```python
from build123d import *

# Parameters (mm, degrees)
SKETCH1_W           = 6.3
SKETCH1_H           = 8
SKETCH1_R           = 1.75
BOSS_EXTRUDE1_DEPTH = 10
SKETCH2_W           = 20
SKETCH2_H           = 6.3
SKETCH2_R           = 1.75
BOSS_EXTRUDE2_DEPTH = 12.15
SKETCH3_R           = 1.325
CUT_EXTRUDE1_DEPTH  = 31.009081959
SKETCH4_W           = 8.6
SKETCH4_H           = 6.3
CUT_EXTRUDE2_DEPTH  = 10
CUT_EXTRUDE3_DEPTH  = 31.009081959
SKETCH13_W          = 5.8
SKETCH13_H          = 3
CUT_EXTRUDE4_DEPTH  = 26.106025173


with BuildPart() as part:
    # Sketch1 → Boss-Extrude1 (new body)
    with BuildSketch(Plane(origin=(0, 0, 0), x_dir=(0, 1, 0), z_dir=(0, 0, 1))):
        Rectangle(SKETCH1_W, SKETCH1_H)
        with Locations(Location((0, 0, 0), (0, 0, 270))):
            Circle(SKETCH1_R, mode=Mode.SUBTRACT)
    extrude(amount=BOSS_EXTRUDE1_DEPTH)

    # Sketch2 → Boss-Extrude2 (add)
    with BuildSketch(Plane.XY.offset(10)):
        Rectangle(SKETCH2_W, SKETCH2_H)
        Circle(SKETCH2_R, mode=Mode.SUBTRACT)
    extrude(amount=BOSS_EXTRUDE2_DEPTH)

    # Sketch3 → Cut-Extrude1 (cut, through all)
    with BuildSketch(Plane(origin=(-10, 0, 0), x_dir=(0, -1, 0), z_dir=(-1, 0, 0))):
        with Locations(Location((0, 19, 0), (0, 0, 90))):
            Circle(SKETCH3_R)
    extrude(amount=-CUT_EXTRUDE1_DEPTH, mode=Mode.SUBTRACT)

    # Sketch4 → Cut-Extrude2 (cut)
    with BuildSketch(Plane.XY.offset(22.15)):
        Rectangle(SKETCH4_W, SKETCH4_H)
    extrude(amount=-CUT_EXTRUDE2_DEPTH, mode=Mode.SUBTRACT)

    # Sketch11 → Cut-Extrude3 (cut, through all)
    with BuildSketch(Plane(origin=(-10, 0, 0), x_dir=(0, -1, 0), z_dir=(-1, 0, 0))):
        with BuildLine():
            Line((-3.15, 19), (-3.15, 24.112369899))
            Line((-3.15, 24.112369899), (3.15, 24.112369899))
            Line((3.15, 24.112369899), (3.15, 19))
            ThreePointArc((3.15, 19), (0, 22.15), (-3.15, 19))
        make_face()
    extrude(amount=-CUT_EXTRUDE3_DEPTH, mode=Mode.SUBTRACT)

    # Sketch13 → Cut-Extrude4 (cut, through all)
    with BuildSketch(Plane(origin=(0, 3.15, 0), x_dir=(-1, 0, 0), z_dir=(0, 1, 0))):
        with Locations((0, 3)):
            Rectangle(SKETCH13_W, SKETCH13_H)
    extrude(amount=-CUT_EXTRUDE4_DEPTH, mode=Mode.SUBTRACT)


solid = part.part
```
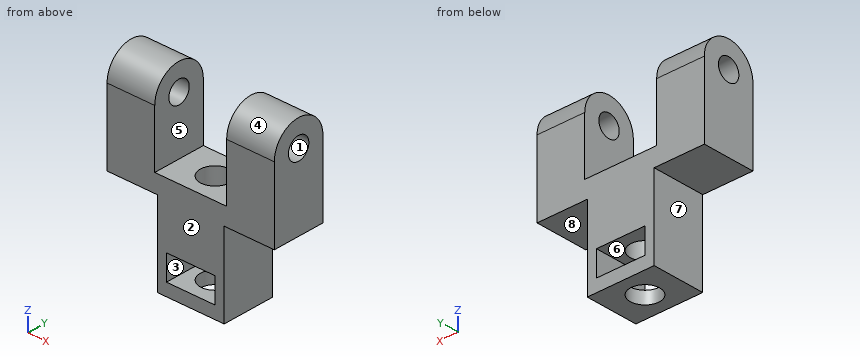
For this review, take the finished solid that the model builds, in its own axes (mm). Face numbers are marked on the shaded views. A direction names the side the tool comes from. Round coordinates to 2 decimals unless told otherwise and drop trailing zeros. Write each loop counter-clockwise with the first axis right and the second up, starting at its lowest first coordinate (ties: lowest second). Pieces come first, ordered by that corner, then holes. Notation, with made-up numbers: (7, 62.25) -> (28, 62.25) arc R27 ccw to (28, 79.25) -> close; hole circle Ø11 at (20.5, -11). An arc over 180 degrees is marked (long way). Use one line per item in the form item = value.
Q1. The part is to be moulded in two halves that separate along Y. For the marked faces 1, 2, 3 and 4, say which applies: released by +Y, released by -Y, zero draft, split by the parting line, or undercut.
Resolved:
face_1 = undercut
face_2 = released by -Y
face_3 = zero draft
face_4 = split by the parting line
Q2. Consider section C-C (x = 0). State the section outline as (y, z) points, then the cut area to 3 significant figures.
Resolved:
outline = (-3.15, 0) -> (-1.75, 0) -> (-1.75, 1.5) -> (-3.15, 1.5) -> close; (-3.15, 4.5) -> (-1.75, 4.5) -> (-1.75, 12.15) -> (-3.15, 12.15) -> close; (1.75, 0) -> (3.15, 0) -> (3.15, 1.5) -> (1.75, 1.5) -> close; (1.75, 4.5) -> (3.15, 4.5) -> (3.15, 12.15) -> (1.75, 12.15) -> close
area = 25.6 mm²
Q3. Consider section D-D (z = 8). State the section outline as (x, y) points, then the cut area to 3 significant figures.
Resolved:
outline = (-4, -3.15) -> (4, -3.15) -> (4, 3.15) -> (-4, 3.15) -> close; hole circle Ø3.5 at (0, 0)
area = 40.8 mm²
Q4. Clearance check with flat-ended pins moving along their axes: pin 1 Ø1.7 at (x, y) = (1, 0) entering from +Z; pin 2 Ø3 at (y, z) = (-1, 4) entering from -X; pin 3 Ø1.8 at (x, y) = (6.5, 1) entering from -Z. State where each tip first meets the part, or that it passes through.
Resolved:
pin_1 = 12.15
pin_2 = -4
pin_3 = 10
Q5. Consider section B-B (x = -2.25). State the section outline as (y, z) points, then the cut area to 3 significant figures.
Resolved:
outline = (-3.15, 0) -> (3.15, 0) -> (3.15, 1.5) -> (-3.15, 1.5) -> close; (-3.15, 4.5) -> (3.15, 4.5) -> (3.15, 12.15) -> (-3.15, 12.15) -> close
area = 57.6 mm²
Q6. Consider section A-A (z = 1.75). State the section outline as (x, y) points.
Resolved:
outline = (-4, -3.15) -> (-2.9, -3.15) -> (-2.9, 3.15) -> (-4, 3.15) -> close; (2.9, -3.15) -> (4, -3.15) -> (4, 3.15) -> (2.9, 3.15) -> close
Q7. To check wall thickness, follow probe 1 along X at (y, z) = (1.25, 3); probe 2 along X at (y, z) = (0, 0.7); probe 3 along Z at (x, y) = (2.75, -0.5). State the ranges of each line that lie inside material, in increasing order. Write a range as from..to.
Resolved:
probe_1 = -4..-2.9, 2.9..4
probe_2 = -4..-1.75, 1.75..4
probe_3 = 0..1.5, 4.5..12.15
Q8. Machinability: for the marked faces 5, 6, 7 and 8, which of the approach directions +Z, -Z, +X, -X, +Y, -Y give a long, thin tool a straight path to every point of the face, cutting with its end or side? Answer none if there is none.
Resolved:
face_5 = +Z, +Y, -Y
face_6 = +Y, -Y
face_7 = -Z, -X, +Y, -Y
face_8 = -Z, +X, +Y, -Y
